```python
from build123d import *

# Parameters (mm, degrees)
SKETCH052_W             = 8.3
SKETCH052_H             = 3.35
PAD022_DEPTH            = 4.55
SKETCH053_W             = 0.6
SKETCH053_H             = 3.35
PAD023_DEPTH            = 0.6
SKETCH054_W             = 7.4
SKETCH054_H             = 2.45
POCKET006_DEPTH         = 3.9
SKETCH055_W             = 6.9
SKETCH055_H             = 1.85
POCKET007_DEPTH         = 0.45
SKETCH004_W             = 0.6
SKETCH004_H             = 0.6
PAD024_DEPTH            = 2.5
SKETCH005_W             = 0.6
SKETCH005_H             = 0.6
PAD025_DEPTH            = 3.75
BODY002_PLACEMENT_ANGLE = 45


with BuildPart() as part:
    # Sketch052 → Pad022 (new body)
    with BuildSketch(Plane.XY):
        with Locations((4.15, 1.675)):
            Rectangle(SKETCH052_W, SKETCH052_H)
    extrude(amount=PAD022_DEPTH)

    # Sketch053 (on Face5 of Pad022) → Pad023 (join)
    with BuildSketch(Plane(origin=(0, 0, 0), x_dir=(1, 0, 0), z_dir=(0, 0, -1))):
        with Locations((0.3, -1.675)):
            Rectangle(SKETCH053_W, SKETCH053_H)
        with Locations((8, -1.675)):
            Rectangle(SKETCH053_W, SKETCH053_H)
    extrude(amount=PAD023_DEPTH)

    # Sketch054 (on Face7 of Pad023) → Pocket006 (cut)
    with BuildSketch(Plane.XY.offset(4.55)):
        with Locations((4.15, 1.675)):
            Rectangle(SKETCH054_W, SKETCH054_H)
    extrude(amount=-POCKET006_DEPTH, mode=Mode.SUBTRACT)

    # Sketch055 (on Face1 of Pocket006) → Pocket007 (cut)
    with BuildSketch(Plane.XZ):
        with Locations((4.15, 3.625)):
            Rectangle(SKETCH055_W, SKETCH055_H)
    extrude(amount=-POCKET007_DEPTH, mode=Mode.SUBTRACT)

    # Sketch004 (on Face3 of Pocket007) → Pad024 (join)
    with BuildSketch(Plane(origin=(0, 0, 0), x_dir=(1, 0, 0), z_dir=(0, 0, -1))):
        with Locations((1.76363, -2.15)):
            Rectangle(SKETCH004_W, SKETCH004_H)
        with Locations((3.01363, -2.15)):
            Rectangle(SKETCH004_W, SKETCH004_H)
        with Locations((4.26363, -2.15)):
            Rectangle(SKETCH004_W, SKETCH004_H)
        with Locations((5.51363, -2.15)):
            Rectangle(SKETCH004_W, SKETCH004_H)
        with Locations((6.76363, -2.15)):
            Rectangle(SKETCH004_W, SKETCH004_H)
    extrude(amount=PAD024_DEPTH)

    # Sketch005 (on Face3 of Pad024) → Pad025 (join)
    with BuildSketch(Plane(origin=(0, 0, 0), x_dir=(1, 0, 0), z_dir=(0, 0, -1))):
        with Locations((1.76363, -2.15)):
            Rectangle(SKETCH005_W, SKETCH005_H)
        with Locations((3.01363, -2.15)):
            Rectangle(SKETCH005_W, SKETCH005_H)
        with Locations((4.26363, -2.15)):
            Rectangle(SKETCH005_W, SKETCH005_H)
        with Locations((5.51363, -2.15)):
            Rectangle(SKETCH005_W, SKETCH005_H)
        with Locations((6.76363, -2.15)):
            Rectangle(SKETCH005_W, SKETCH005_H)
    extrude(amount=-PAD025_DEPTH)


with BuildPart() as part_1:
    # Body002 placement: moved
    add(part.part.moved(Location((41.05, -48.95, 120))).rotate(Axis((41.05, -48.95, 120), (0, 0, 1)), BODY002_PLACEMENT_ANGLE))


solid = part_1.part
```
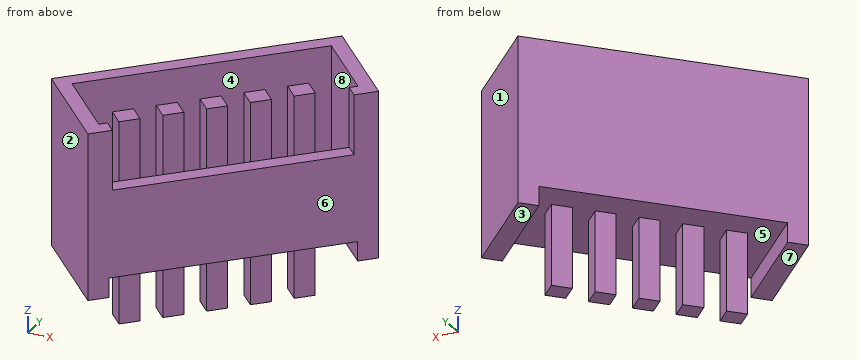
The model under review builds one solid part; all positions refer to its coordinate system, in mm. Face numbers are marked on the shaded views. A direction names the side the tool comes from. Coordinates: 2 decimals unless noted, no trailing zeros. Write each loop counter-clockwise with the first axis right and the second up, starting at its lowest first coordinate (ties: lowest second). Pieces come first, ordered by that corner, then holes. Notation, with made-up numbers: (48, 68.25) - (73, 68.25) arc R32 ccw to (73, 106.25) - close; hole circle Ø2 at (14.5, -6). An arc over 180 degrees is marked (long way). Answer in a Markdown table with one row per item. Add a question column.
Q1. Consider section B-B on z = 123.5. Give the number of separate pieces and of enclosed holes in the cut face, then the cut area to 3 significant figures.
Q2. To check wall thickness, follow line 1 along X through (y, z) = (-45.5, 121); line 2 along Y through (x, z) = (44, 121.5); line 3 along Y through (x, z) = (41.5, 121.25). State the ranges of each line that lie inside material, in increasing order. Write a range as from..to.
Q3. For the marked faces 1, 2, 3, 4 and 5, list the 3-axis set-ups (+Z, -Z, +X, -X, +Y, -Y) from which the entire face can be reached by the end or side of a thin tool; tool diameter is ignored.
Q4. Consider section A-A on z = 119.75. Give the boundary of the cut face in (x, y), then the cut area to 3 significant figures.
Q5. Draft analysis for pull direction Y (two halves, no side actions). For the marked faces 6, 7 and 8, state which applies: +Y half, -Y half, draft (parallel to the pull), parting line (faces both ways), or undercut.
Q6. Consider section D-D on z = 121.5. Give the boundary of the cut face in (x, y), then the cut area to 3 significant figures.
Q7. Clearance check with flat-ended pins moving along their axes: pin 1 (0.9 mm diameter, centred on x = 44.5, y = -42.5, fed in from +Z); pin 2 (2.5 mm diameter, centred on x = 44, y = -46, fed in from +Z); pin 3 (1 mm diameter, centred on x = 42.5, z = 123.5, fed in from -Y). State where each tip first meets the part, or that it passes through.
Q8. Consider section C-C on z = 118.5. Give the boundary of the cut face in (x, y), then the cut area to 3 significant figures.
Answers below:
| question | item | result |
|---|---|---|
| 1 | separate pieces | 6 |
| 1 | enclosed holes | 0 |
| 1 | area | 8.37 mm² |
| 2 | line 1 | 39.76..40.4, 41.44..41.88, 43.86..44.5 |
| 2 | line 2 | -46..-45.36, -42.76..-42.54, -41.9..-41.26 |
| 2 | line 3 | -48.5..-47.86, -45.56..-45.04, -44.4..-43.76 |
| 3 | face 1 | +Z, -Z, +X, +Y |
| 3 | face 2 | +Z, -Z, -X, -Y |
| 3 | face 3 | -Z, +X, +Y |
| 3 | face 4 | +Z |
| 3 | face 5 | -Z |
| 4 | outline | (38.68, -46.58) - (41.05, -48.95) - (41.47, -48.53) - (39.11, -46.16) - close; (40.35, -46.18) - (40.78, -46.61) - (41.2, -46.18) - (40.78, -45.76) - close; (41.24, -45.3) - (41.66, -45.72) - (42.08, -45.3) - (41.66, -44.87) - close; (42.12, -44.41) - (42.54, -44.84) - (42.97, -44.41) - (42.54, -43.99) - close; (43, -43.53) - (43.43, -43.96) - (43.85, -43.53) - (43.43, -43.11) - close; (43.89, -42.65) - (44.31, -43.07) - (44.74, -42.65) - (44.31, -42.22) - close; (44.13, -41.14) - (46.49, -43.51) - (46.92, -43.08) - (44.55, -40.71) - close |
| 4 | area | 5.82 mm² |
| 5 | face 6 | -Y half |
| 5 | face 7 | draft |
| 5 | face 8 | undercut |
| 6 | outline | (38.68, -46.58) - (41.05, -48.95) - (46.92, -43.08) - (44.55, -40.71) - close; (40.35, -46.18) - (40.78, -46.61) - (41.2, -46.18) - (40.78, -45.76) - close; (41.24, -45.3) - (41.66, -45.72) - (42.08, -45.3) - (41.66, -44.87) - close; (42.12, -44.41) - (42.54, -44.84) - (42.97, -44.41) - (42.54, -43.99) - close; (43, -43.53) - (43.43, -43.96) - (43.85, -43.53) - (43.43, -43.11) - close; (43.89, -42.65) - (44.31, -43.07) - (44.74, -42.65) - (44.31, -42.22) - close; hole (39.32, -46.58) - (41.05, -48.31) - (46.28, -43.08) - (44.55, -41.35) - close |
| 6 | area | 11.5 mm² |
| 7 | pin 1 | z = 123.75 |
| 7 | pin 2 | z = 122.7 |
| 7 | pin 3 | y = -45.38 |
| 8 | outline | (40.35, -46.18) - (40.78, -46.61) - (41.2, -46.18) - (40.78, -45.76) - close; (41.24, -45.3) - (41.66, -45.72) - (42.08, -45.3) - (41.66, -44.87) - close; (42.12, -44.41) - (42.54, -44.84) - (42.97, -44.41) - (42.54, -43.99) - close; (43, -43.53) - (43.43, -43.96) - (43.85, -43.53) - (43.43, -43.11) - close; (43.89, -42.65) - (44.31, -43.07) - (44.74, -42.65) - (44.31, -42.22) - close |
| 8 | area | 1.80 mm² |
